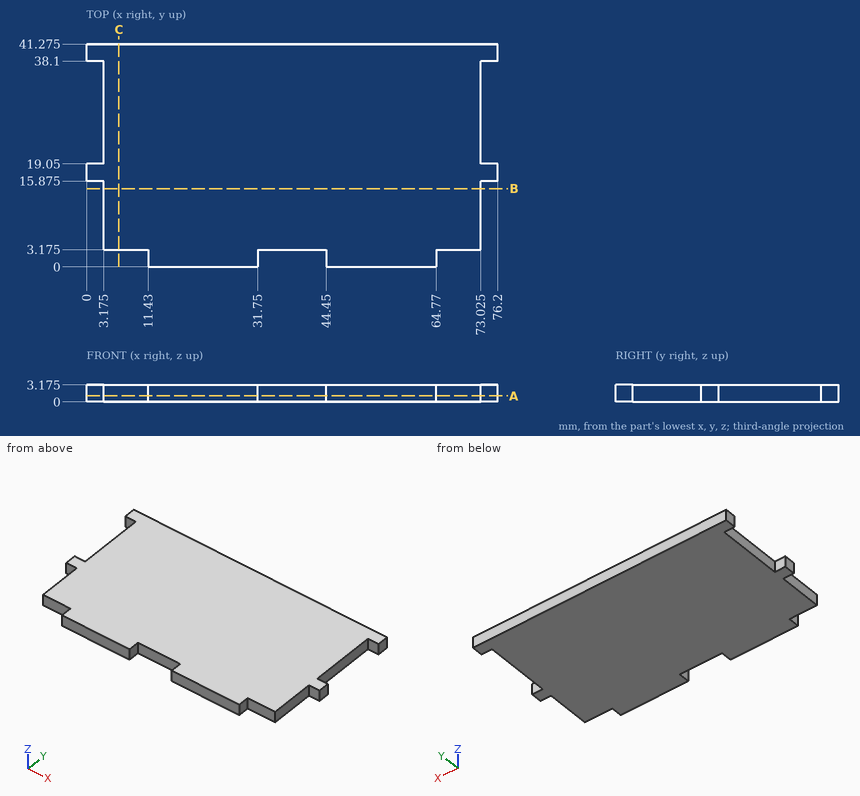
Part print with two shaded views. Sizes in mm from the minimum x, y, z corner. Coordinates: 2 decimals unless noted, no trailing zeros. Loops run counter-clockwise (first coordinate to the right, second up) from the corner with the lowest first, then second, coordinate; pieces in that order, holes last. Notation, with made-up numbers: M 32,20 L 68,20 A18 ccw 68,25 Z; hole C -3,-2 d8. An arc over 180 degrees is marked long. Use CSV: the item, a comma, the result in double quotes. Start each with the question number.
1. Band-saw the part on C-C, the plane x = 6. List the corners of the cut face in (y, z) (3 decimals), then the cut area to 3 significant figures.
2. Band-saw the part on A-A, the plane z = 1.1. List the corners of the cut face in (x, y) (3 decimals).
3. Band-saw the part on B-B, the plane y = 14.5. List the corners of the cut face in (x, z) (3 decimals).
4. Probe probe 1 along X at (y, z) = (22, 0.65) (3 decimals); probe 2 along Y at (x, z) = (38, 2.7) (3 decimals). List the from-to ranges inside material, lowest first. Write a range as [from, to].
5. Flat gauge pins, fed straight in: pin 1 (1.5 mm diameter, centred on y = 31.5, z = 2, fed in from +X) (3 decimals); pin 2 (1 mm diameter, centred on y = 1, z = 2, fed in from +X); pin 3 (1 mm diameter, centred on x = 1, z = 1.5, fed in from -Y) (3 decimals). Where does each tip first touch, or does it go through?
Entries:
1,outline,"M 3.175,0 L 41.275,0 L 41.275,3.175 L 3.175,3.175 Z"
1,area,"121 mm2"
2,outline,"M 0,15.875 L 3.175,15.875 L 3.175,3.175 L 11.43,3.175 L 11.43,0 L 31.75,0 L 31.75,3.175 L 44.45,3.175 L 44.45,0 L 64.77,0 L 64.77,3.175 L 73.025,3.175 L 73.025,15.875 L 76.2,15.875 L 76.2,19.05 L 73.025,19.05 L 73.025,38.1 L 76.2,38.1 L 76.2,41.275 L 0,41.275 L 0,38.1 L 3.175,38.1 L 3.175,19.05 L 0,19.05 Z"
3,outline,"M 3.175,0 L 73.025,0 L 73.025,3.175 L 3.175,3.175 Z"
4,probe 1,"x = [3.175, 73.025]"
4,probe 2,"y = [3.175, 41.275]"
5,pin 1,"stops at x = 73.025"
5,pin 2,"stops at x = 64.77"
5,pin 3,"stops at y = 15.875"
